from build123d import *

# Parameters (mm, degrees)
EXTRUDE_1_DEPTH     = 100
CUT_EXTRUDE_1_DEPTH = 849.335356313
CUT_EXTRUDE_2_DEPTH = 849.335356313
CUT_EXTRUDE_3_REACH = 850.335


with BuildPart() as part:
    # 草图1 → 凸台-拉伸1 (new body)
    with BuildSketch(Plane.XY):
        with BuildLine():
            Line((670, 0), (830, 0))
            ThreePointArc((830, 0), (826.841599416, -72.339266481), (817.390435, -144.127987464))
            Line((817.390435, -144.127987464), (659.821194518, -116.344279037))
            ThreePointArc((659.821194518, -116.344279037), (667.450447721, -58.394347641), (670, 0))
        make_face()
    extrude(amount=EXTRUDE_1_DEPTH)

    # 草图3 → 切除-拉伸1 (cut, through all)
    with BuildSketch(Plane.XY.offset(100)):
        with BuildLine():
            Line((778.121311296, -55.529045617), (777.031864512, -67.981479343))
            Line((777.031864512, -67.981479343), (775.942417727, -80.433913069))
            Line((775.942417727, -80.433913069), (825.658378988, -84.783496076))
            ThreePointArc((825.658378988, -84.783496076), (826.841599416, -72.339266481), (827.837272557, -59.878628624))
            Line((827.837272557, -59.878628624), (778.121311296, -55.529045617))
        make_face()
    extrude(amount=-CUT_EXTRUDE_1_DEPTH, mode=Mode.SUBTRACT)

    # 草图5 → 切除-旋转1 (revolve, cut)
    with BuildSketch(Plane(origin=(-3.050450996, -34.866814433, 0), x_dir=(-0.9961946980917455, 0.08715574274765771, 0), z_dir=(-0.08715574274765771, -0.9961946980917455, 0)), mode=Mode.PRIVATE) as cut_revolve_1_sk:
        Polygon((-805, -100), (-810, -100), (-818.682408883, -50.759612349), (-818.682408883, 0), (-805, 0), align=None)
    cut_revolve_1 = revolve(cut_revolve_1_sk.sketch.rotate(Axis((798.886280968, -105.027187345, 0), (0, 0, 1)), 185), axis=Axis((798.886280968, -105.027187345, 0), (0, 0, 1)), mode=Mode.SUBTRACT)

    # 镜向1: 切除-旋转1 across plane
    add(cut_revolve_1.mirror(Plane(origin=(0, 0, 0), x_dir=(0, 0, 1), z_dir=(-0.08715574274765854, -0.9961946980917457, 0))), mode=Mode.SUBTRACT)

    # 草图6 → 切除-拉伸2 (cut, through all)
    with BuildSketch(Plane(origin=(0, 0, 0), x_dir=(-1, 0, 0), z_dir=(0, 0, -1))):
        with BuildLine():
            Line((-669.669272048, -118.080760814), (-694.289465874, -122.421965255))
            ThreePointArc((-694.289465874, -122.421965255), (-695.331349084, -116.358562132), (-696.32028012, -110.286297853))
            Line((-696.32028012, -110.286297853), (-671.628071605, -106.375436227))
            ThreePointArc((-671.628071605, -106.375436227), (-670.674209045, -112.232371985), (-669.669272048, -118.080760814))
        make_face()
        with BuildLine():
            Line((-679.896432706, -11.867636377), (-704.892625085, -12.303946538))
            ThreePointArc((-704.892625085, -12.303946538), (-704.97315576, -6.152207526), (-705, 0))
            Line((-705, 0), (-680, 0))
            ThreePointArc((-680, 0), (-679.974107684, -5.934044139), (-679.896432706, -11.867636377))
        make_face()
    extrude(amount=-CUT_EXTRUDE_2_DEPTH, mode=Mode.SUBTRACT)

    # 草图7 → 切除-拉伸3 (cut, up to next)
    with BuildSketch(Plane.XY.offset(100), mode=Mode.PRIVATE) as cut_extrude_3_sk1:
        with BuildLine():
            Line((767.5, 0), (829.459141918, -29.958836576))
            ThreePointArc((829.459141918, -29.958836576), (829.864774464, -14.981859167), (830, 0))
            Line((830, 0), (767.5, 0))
        make_face()
    cut_extrude_3_tool1 = extrude(cut_extrude_3_sk1.sketch, amount=-CUT_EXTRUDE_3_REACH, mode=Mode.PRIVATE) & part.part
    # 草图7 → 切除-拉伸3 (cut, up to next)
    with BuildSketch(Plane.XY.offset(100), mode=Mode.PRIVATE) as cut_extrude_3_sk2:
        with BuildLine():
            Line((822.060091144, -114.530373912), (755.839950437, -133.274976359))
            Line((755.839950437, -133.274976359), (817.390435, -144.127987464))
            ThreePointArc((817.390435, -144.127987464), (819.858836386, -129.350254733), (822.060091144, -114.530373912))
        make_face()
    cut_extrude_3_tool2 = extrude(cut_extrude_3_sk2.sketch, amount=-CUT_EXTRUDE_3_REACH, mode=Mode.PRIVATE) & part.part
    add(cut_extrude_3_tool1.solids().sort_by_distance((809.046215, -10.000647, 100))[0], mode=Mode.SUBTRACT)
    add(cut_extrude_3_tool2.solids().sort_by_distance((798.491579, -130.640686, 100))[0], mode=Mode.SUBTRACT)


solid = part.part
The listing builds one solid part. Answer for the finished solid, in the listing's coordinates (mm). A direction names the side the tool comes from. Coordinates: 2 decimals unless noted, no trailing zeros. Write each loop counter-clockwise with the first axis right and the second up, starting at its lowest first coordinate (ties: lowest second). Pieces come first, ordered by that corner, then holes. Notation, with made-up numbers: (79, 88) - (101, 88) arc R8 ccw to (101, 102) - close; hole circle Ø6 at (63, 1.25). An arc over 180 degrees is marked (long way). Return JSON: item names as keys, results as strings.
1. For a pull along X with two mould halves and no side action, classify faces 1 (the face through (704.972, -6.238, 49.3)), 2 (the face through (667.38, -59.21, 49.3)), 3 (the face through (800.45, -82.58, 50.7)) as +X half, -X half, draft (parallel to the pull), parting line (faces both ways), or undercut.
Final values:
{"face 1": "undercut", "face 2": "-X half", "face 3": "+X half"}
2. Consider line 1 along Y through (x, z) = (817.5, 47.5); line 2 along X through (y, z) = (-30, 77.5); line 3 along Y through (x, z) = (793.5, 14). Determine where each line is inside the solid, lowest interval first.
Final values:
{"line 1": "-115.82 to -84.07, -58.97 to -40.83, -29.76 to -24.18", "line 2": "669.33 to 797.75, 812.23 to 829.46", "line 3": "-122.61 to -117.6, -92.45 to -81.97, -56.87 to -42.73, -27.86 to -12.57"}
3. Each of these flat-tipped pins is pushed along its axis until it touches: pin 1 Ø5 at (y, z) = (-39.5, 87) entering from -X; pin 2 Ø3 at (y, z) = (-113, 58.5) entering from +X; pin 3 Ø10 at (y, z) = (-101.5, 72) entering from +X. Where does it stop, or does it pass through?
Final values:
{"pin 1": "x = 668.68", "pin 2": "x = 822.48", "pin 3": "x = 824.37"}
4. Which of the six approach directions +Z, -Z, +X, -X, +Y, -Y give full straight-line access (tool end or side, diameter ignored) to faces 4 (the face through (814.23, -45.38, 25.02)), 5 (the face through (824.02, -99.46, 49.3)), 6 (the face through (695.317, -116.444, 49.3))?
Final values:
{"face 4": "-Z", "face 5": "+Z, -Z, +X, -Y", "face 6": "+Z, -Z"}
5. The part is cut by section B-B on x = 771. Determine the outline of the cut face in (y, z), then the cut area to 3 significant figures.
Final values:
{"outline": "(-128.98, 0) - (-1.69, 0) - (-1.69, 100) - (-128.98, 100) - close", "area": "12,700 mm^2"}
6. The part is cut by section A-A on z = 9. Determine the outline of the cut face in (x, y), then the cut area to 3 significant figures.
Final values:
{"outline": "(659.82, -116.34) - (669.67, -118.08) arc R680 ccw to (671.63, -106.38) - (696.32, -110.29) arc R705 cw to (694.29, -122.42) - (755.84, -133.27) - (822.06, -114.53) arc R830 ccw to (825.66, -84.78) - (775.94, -80.43) - (778.12, -55.53) - (827.84, -59.88) arc R830 ccw to (829.46, -29.96) - (767.5, 0) - (705, 0) arc R705 cw to (704.89, -12.3) - (679.9, -11.87) arc R680 ccw to (680, 0) - (670, 0) arc R670 cw to start; hole circle Ø27.36 at (798.89, -105.03); hole circle Ø27.36 at (804.99, -35.29)", "area": "16,000 mm^2"}
7. The part is cut by section C-C on y = -73. Determine the outline of the cut face in (x, z), then the cut area to 3 significant figures.
Final values:
{"outline": "(666.01, 0) - (776.59, 0) - (776.59, 100) - (666.01, 100) - close", "area": "11,100 mm^2"}
